Geometry: final body of the model. Coordinates: model frame, mm. Give positions to 0.01 mm unless a question says otherwise; leave off trailing zeros. Loops run counter-clockwise (first coordinate to the right, second up) from the corner with the lowest first, then second, coordinate; pieces in that order, holes last. Notation, with made-up numbers: (9, 2.5) -> (61, 2.5) arc R18 ccw to (61, 6.5) -> close; hole circle Ø8 at (88.5, 37). An arc over 180 degrees is marked (long way). One line per question, with ' | ' between items. Start each with the question number.
Item 1: Section C-C on z = 0. Return loops of the section in (x, y), then the cut area to 3 significant figures.
Item 2: Section B-B on y = 7.5. Return loops of the section in (x, z), then the cut area to 3 significant figures.
Item 3: Material intervals for line 1 along X through (y, z) = (7, -0.1); line 2 along Y through (x, z) = (0.4, 0.1); line 3 along X through (y, z) = (7.75, -0.15), sorted ascending. Write a range as [from, to].
Item 4: Section A-A on x = 0.1. Return loops of the section in (y, z).
from build123d import *

# Parameters (mm, degrees)
SKETCH1_W      = 2.9
SKETCH1_H      = 10
SKETCH1_W_2    = 1.4
SKETCH1_H_2    = 2.5
EXTRUDE1_DEPTH = 0.2
FILLET1_R      = 0.5
FILLET2_R      = 0.6
FILLET3_R      = 0.1


with BuildPart() as part:
    # Sketch1 → Extrude1 (new body, symmetric)
    with BuildSketch(Plane.XY):
        with Locations((0, 5)):
            Rectangle(SKETCH1_W, SKETCH1_H)
        with Locations((0, 7.75)):
            Rectangle(SKETCH1_W_2, SKETCH1_H_2, mode=Mode.SUBTRACT)
    extrude(amount=EXTRUDE1_DEPTH, both=True)

    # Fillet1
    fillet1_edges = [part.edges().sort_by_distance(p)[0] for p in [
        (-0.7, 9, 0),
        (-0.7, 6.5, 0),
        (0.7, 6.5, 0),
        (0.7, 9, 0),
    ]]
    fillet(fillet1_edges, radius=FILLET1_R)

    # Fillet2
    fillet2_edges = [part.edges().sort_by_distance(p)[0] for p in [
        (-1.45, 10, 0),
        (1.45, 10, 0),
    ]]
    fillet(fillet2_edges, radius=FILLET2_R)

    # Fillet3
    fillet3_edges = [part.edges().sort_by_distance(p)[0] for p in [
        (1.45, 4.7, 0.2),
        (0, 6.5, -0.2),
        (0, 6.5, 0.2),
        (0.7, 7.75, -0.2),
        (0.7, 7.75, 0.2),
        (0, 9, -0.2),
        (0, 9, 0.2),
        (-0.7, 7.75, -0.2),
        (-0.7, 7.75, 0.2),
        (0.553553391, 6.646446609, -0.2),
        (0.553553391, 6.646446609, 0.2),
        (0.553553391, 8.853553391, -0.2),
        (0.553553391, 8.853553391, 0.2),
        (-0.553553391, 8.853553391, -0.2),
        (-0.553553391, 8.853553391, 0.2),
        (-0.553553391, 6.646446609, -0.2),
        (-0.553553391, 6.646446609, 0.2),
        (1.45, 4.7, -0.2),
        (0, 10, -0.2),
        (0, 10, 0.2),
        (-1.45, 4.7, -0.2),
        (-1.274264069, 9.824264069, -0.2),
        (1.274264069, 9.824264069, -0.2),
        (-1.45, 4.7, 0.2),
        (-1.274264069, 9.824264069, 0.2),
        (1.274264069, 9.824264069, 0.2),
    ]]
    fillet(fillet3_edges, radius=FILLET3_R)


solid = part.part
Result sheet:
1) outline: (-1.45, 0) -> (1.45, 0) -> (1.45, 9.4) arc R0.6 ccw to (0.85, 10) -> (-0.85, 10) arc R0.6 ccw to (-1.45, 9.4) -> close; hole (-0.7, 7) arc R0.5 ccw to (-0.2, 6.5) -> (0.2, 6.5) arc R0.5 ccw to (0.7, 7) -> (0.7, 8.5) arc R0.5 ccw to (0.2, 9) -> (-0.2, 9) arc R0.5 ccw to (-0.7, 8.5) -> close | area: 25.6 mm²
2) outline: (-1.45, -0.1) arc R0.1 ccw to (-1.35, -0.2) -> (-0.8, -0.2) arc R0.1 ccw to (-0.7, -0.1) -> (-0.7, 0.1) arc R0.1 ccw to (-0.8, 0.2) -> (-1.35, 0.2) arc R0.1 ccw to (-1.45, 0.1) -> close; (0.7, -0.1) arc R0.1 ccw to (0.8, -0.2) -> (1.35, -0.2) arc R0.1 ccw to (1.45, -0.1) -> (1.45, 0.1) arc R0.1 ccw to (1.35, 0.2) -> (0.8, 0.2) arc R0.1 ccw to (0.7, 0.1) -> close | area: 0.583 mm²
3) line 1: x = [-1.45, -0.7], [0.7, 1.45] | line 2: y = [0, 6.54], [8.96, 10] | line 3: x = [-1.44, -0.71], [0.71, 1.44]
4) outline: (0, -0.2) -> (6.4, -0.2) arc R0.1 ccw to (6.5, -0.1) -> (6.5, 0.1) arc R0.1 ccw to (6.4, 0.2) -> (0, 0.2) -> close; (9, -0.1) arc R0.1 ccw to (9.1, -0.2) -> (9.9, -0.2) arc R0.1 ccw to (10, -0.1) -> (10, 0.1) arc R0.1 ccw to (9.9, 0.2) -> (9.1, 0.2) arc R0.1 ccw to (9, 0.1) -> close
